Design review of the part built by this model. Coordinates are the model's own, in mm. A direction names the side the tool comes from. Coordinates: 2 decimals unless noted, no trailing zeros. Loops run counter-clockwise (first coordinate to the right, second up) from the corner with the lowest first, then second, coordinate; pieces in that order, holes last. Notation, with made-up numbers: (35.5, 31) -> (55.5, 31) arc R30 cw to (55.5, 67) -> close; hole circle Ø1 at (15.25, 73). An arc over 180 degrees is marked (long way). Answer as a JSON object with one key per item and string values.
```python
from build123d import *

# Parameters (mm, degrees)
F0_W     = 16
F0_H     = 12
F0_R     = 1.8
F1_DEPTH = 13
F2_W     = 16
F2_H     = 10
F2_R     = 1.8
F3_DEPTH = 3
F5_DEPTH = 16.001
F6_R     = 1.3
F7_DEPTH = 10


# Not quite as in the source:
# - a feature names something its author has since deleted; it is built from what else it names


with BuildPart() as f1:
    # F0 (on Front) → F1 (new body)
    with BuildSketch(Plane.XZ):
        with Locations((-5.3398377105, -1)):
            Rectangle(F0_W, F0_H)
        with Locations((-10.3398377105, 0)):
            Circle(F0_R, mode=Mode.SUBTRACT)
    extrude(amount=F1_DEPTH)

    # F2 (on face) → F3 (cut)
    with BuildSketch(Plane.XZ.offset(13)):
        with Locations((-5.3398377105, 0)):
            Rectangle(F2_W, F2_H)
        with Locations((-10.3398377105, 0)):
            Circle(F2_R, mode=Mode.SUBTRACT)
    extrude(amount=-F3_DEPTH, mode=Mode.SUBTRACT)

    # F4 (on face) → F5 (cut, through all)
    with BuildSketch(Plane.YZ.offset(2.6601622895)):
        with BuildLine():
            ThreePointArc((-2.3, 2.3), (-0.6736544033, 1.6263455967), (0, 0))
            Line((0, 0), (0, 5))
            Line((0, 5), (-10, 5))
            Line((-10, 5), (-2.3, 2.3))
        make_face()
        with BuildLine():
            Line((0, -7), (0, 0))
            ThreePointArc((0, 0), (-0.6736544033, -1.6263455967), (-2.3, -2.3))
            Line((-2.3, -2.3), (-10, -7))
            Line((-10, -7), (0, -7))
        make_face()
    extrude(amount=-F5_DEPTH, mode=Mode.SUBTRACT)

    # F6 (on face) → F7 (cut)
    with BuildSketch(Plane.YZ.offset(2.6601622895)):
        with Locations((-2.3, 0)):
            Circle(F6_R)
    extrude(amount=-F7_DEPTH, mode=Mode.SUBTRACT)


solid = f1.part
```
1) The part is to be moulded in two halves that separate along Y. For faces 1 (the flat face through (-5.228, -6.204, 3.669)), 2 (the flat face through (-5, -11, -7)), 3 (the cylindrical face through (-2, -1, 0)), say which applies: pulls with the +Y half, pulls with the -Y half, needs draft (parallel to the pull), parting line crosses it, or undercut.
Completed:
{"face 1": "pulls with the +Y half", "face 2": "needs draft", "face 3": "undercut"}
2) For faces 4 (the flat face through (-5, -12, -5)), 5 (the flat face through (-5.23, -6.1, -4.62)), 6 (the flat face through (-7.34, -2, 0)), list the 3-axis set-ups (+Z, -Z, +X, -X, +Y, -Y) from which the entire face can be reached by the end or side of a thin tool; tool diameter is ignored.
Completed:
{"face 4": "+Z, +X, -X, -Y", "face 5": "-Z, +X, -X, +Y", "face 6": "+X"}
3) Clearance check with flat-ended pins moving along their axes: pin 1 Ø5 at (x, y) = (-0.5, -2) entering from +Z; pin 2 Ø2.5 at (y, z) = (-2.3, 0) entering from +X; pin 3 Ø3 at (x, z) = (-10.34, 0) entering from +Y. State where each tip first meets the part, or that it passes through.
Completed:
{"pin 1": "z = 3.07", "pin 2": "x = -7.34", "pin 3": "through"}
4) Wall thickness on probe 1 along Z at (x, y) = (-1.25, -2.3); probe 2 along Z at (x, y) = (-6, -2.5); probe 3 along X at (y, z) = (-8, 1.5): over which ranges is each line inside the solid? List them lowest first.
Completed:
{"probe 1": "-2.3 to -1.3, 1.3 to 2.3", "probe 2": "-2.42 to -1.28, 1.28 to 2.37", "probe 3": "-13.34 to -11.33, -9.34 to 2.66"}
5) Add section B-B, the plane z = 0.75. Give the boundary of the cut face in (x, y).
Completed:
{"outline": "(-13.34, -10) -> (-11.98, -10) -> (-11.98, -0.13) -> (-13.34, -0.13) -> close; (-8.7, -10) -> (2.66, -10) -> (2.66, -3.36) -> (-7.34, -3.36) -> (-7.34, -1.24) -> (2.66, -1.24) -> (2.66, -0.13) -> (-8.7, -0.13) -> close"}
6) Add section C-C, the plane x = -2.75. Give the boundary of the cut face in (y, z).
Completed:
{"outline": "(-13, -7) -> (-10, -7) -> (-2.3, -2.3) arc R2.3 ccw to (-2.3, 2.3) -> (-10, 5) -> (-10, -5) -> (-13, -5) -> close; hole circle Ø2.6 at (-2.3, 0)"}
7) Add section A-A, the plane x = -10.5. Give the boundary of the cut face in (y, z).
Completed:
{"outline": "(-13, -7) -> (-10, -7) -> (-2.3, -2.3) arc R2.3 ccw to (-0.86, -1.79) -> (-10, -1.79) -> (-10, -5) -> (-13, -5) -> close; (-10, 1.79) -> (-0.86, 1.79) arc R2.3 ccw to (-2.3, 2.3) -> (-10, 5) -> close"}
8) Add section D-D, the plane y = -6.75. Give the boundary of the cut face in (x, z), and give its area (3 significant figures).
Completed:
{"outline": "(-13.34, -5.02) -> (2.66, -5.02) -> (2.66, 3.86) -> (-13.34, 3.86) -> close; hole circle Ø3.6 at (-10.34, 0)", "area": "132 mm²"}
